Could you check a few things on this model? Use its own coordinates, in mm. Face numbers are marked on the shaded views. Give positions to 0.01 mm unless a question says otherwise; leave off trailing zeros. Loops run counter-clockwise (first coordinate to the right, second up) from the corner with the lowest first, then second, coordinate; pieces in that order, holes last. Notation, with made-up numbers: M 51,5 L 76,5 A16 cw 76,13 Z; hole C -2,68 d1. An arc over 180 degrees is marked long. Use CSV: the item, a comma, the result in double quotes.
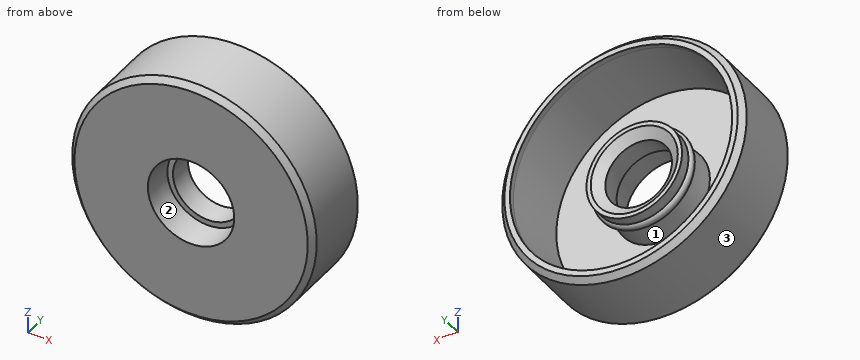
```python
from build123d import *


with BuildPart() as part:
    # 草图1 → 旋转1 (revolve)
    with BuildSketch(Plane.XY):
        with BuildLine():
            Line((-9.518812351, 1), (-4.301871051, 1))
            Line((-4.301871051, 1), (-4.101871051, 3.286010461))
            ThreePointArc((-4.101871051, 3.286010461), (-4.537121231, 3.630475426), (-4.301871051, 4.133224056))
            Line((-4.301871051, 4.133224056), (-4.301871051, 5.071428571))
            Line((-4.301871051, 5.071428571), (-3.918095147, 5.071428571))
            Line((-3.918095147, 5.071428571), (-3, 4.428571429))
            Line((-3, 4.428571429), (-3.168728137, 2.5))
            Line((-3.168728137, 2.5), (-3.668728137, 2.5))
            Line((-3.668728137, 2.5), (-3.887449796, 0))
            Line((-3.887449796, 0), (-10.5, 0))
            Line((-10.5, 0), (-11, 0.5))
            Line((-11, 0.5), (-11, 6.5))
            Line((-11, 6.5), (-10.5, 7))
            Line((-10.5, 7), (-10, 7))
            Line((-10, 7), (-10, 6.5))
            Line((-10, 6.5), (-9.518812351, 1))
        make_face()
    revolve(axis=Axis((0, 5.836193369, 0), (0, -1, 0)))


solid = part.part
```
1. I want a section at C-C, the plane y = 6. List the corners of the cut face in (x, z) for me.
Outcome:
outline,"C 0,0 d22; hole C 0,0 d19.91"
2. If we mould it in two halves opening along Y, with no side actions, what happens to the marked faces 1, 2 and 3? For each: +Y half, -Y half, draft (parallel to the pull), parting line (faces both ways), or undercut.
Outcome:
face 1,"undercut"
face 2,"-Y half"
face 3,"draft"
3. Please list where these lines run through material, in increasing order: line 1 (Z direction, x = -2.5, y = 4.5); line 2 (Y direction, x = 7.75, z = 0); line 3 (X direction, y = 6.75, z = -6.75).
Outcome:
line 1,"-10.71 to -9.5, -3.5 to -1.84, 1.84 to 3.5, 9.5 to 10.71"
line 2,"0 to 1"
line 3,"-8.37 to -7.38, 7.38 to 8.37"
4. I'm going to push flat-ended pins straight in: pin 1 Ø9.5 at (x, z) = (0, -0.5) entering from +Y; pin 2 Ø1.5 at (y, z) = (4, 8.5) entering from +X; pin 3 Ø3 at (x, y) = (-2, 1.5) entering from -Z; pin 4 Ø8 at (x, z) = (5.5, -3) entering from -Y. Where does each tip first touch, or does it pass through?
Outcome:
pin 1,"y = 5.07"
pin 2,"x = 7.81"
pin 3,"z = -10.99"
pin 4,"y = 0"
